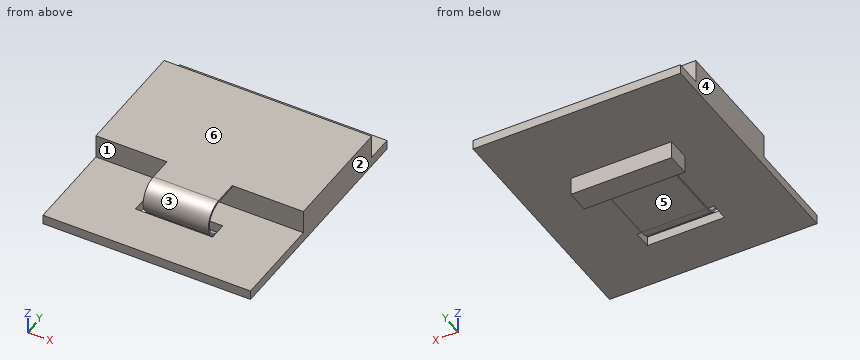
from build123d import *

# Parameters (mm, degrees)
F0_W     = 35
F0_H     = 40
F0_W_2   = 13
F0_H_2   = 3
F1_DEPTH = 1.6
F2_W     = 11
F2_H     = 1
F3_DEPTH = 4
F5_W     = 11
F5_H     = 0.3
F7_W     = 17
F7_H     = 3.9
F8_DEPTH = 3


with BuildPart() as f1:
    # F0 (on Top) → F1 (new body)
    with BuildSketch(Plane.XY):
        Rectangle(F0_W, F0_H)
        with Locations((0, -10.5)):
            Rectangle(F0_W_2, F0_H_2, mode=Mode.SUBTRACT)
    extrude(amount=F1_DEPTH)

    # F2 (on face) → F3 (join)
    with BuildSketch(Plane.XY.offset(1.6)):
        Polygon((17.5, 15.5), (-17.5, 15.5), (-17.5, -4.5), (-5.5, -4.5), (-5.5, -3.5), (5.5, -3.5), (5.5, -4.5), (17.5, -4.5), align=None)
        with Locations((0, -4)):
            Rectangle(F2_W, F2_H)
    extrude(amount=F3_DEPTH)

    # F6: sweep along a path in F4
    with BuildLine(Plane.YZ) as f6_path:
        Line((-4.5, 5.6), (-8.5, 5.6))
        ThreePointArc((-8.5, 5.6), (-11.5, 2.6), (-8.5, -0.4))
        Line((-8.5, -0.4), (6.975, -0.4))
    # F5 (on face) → F6 (sweep)
    with BuildSketch(Plane.XZ.offset(4.5)):
        with Locations((0, 5.45)):
            Rectangle(F5_W, F5_H)
    sweep(path=f6_path.line)

    # F7 (on face) → F8 (join)
    with BuildSketch(Plane(origin=(0, 0, 0), x_dir=(1, 0, 0), z_dir=(0, 0, -1))):
        with Locations((0, -5.025)):
            Rectangle(F7_W, F7_H)
    extrude(amount=F8_DEPTH)


solid = f1.part
Could you check a few things on this model? Use its own coordinates, in mm. Face numbers are marked on the shaded views. A direction names the side the tool comes from. Coordinates: 2 decimals unless noted, no trailing zeros. Order: outer loops, then holes, each group sorted by start corner. A loop starts at its lowest first (then second) coordinate and runs counter-clockwise, first axis right, second up. Notation, with made-up numbers: (23.25, 43) - (30.25, 43) arc R21 ccw to (30.25, 67) - close; hole circle Ø5 at (-13.5, 56). An arc over 180 degrees is marked (long way). Answer in a Markdown table with one row per item. Add a question column.
(1) If we section it at A-A, the plane z = 2.6: Please give me the cut outline in (x, y).
(2) If we section it at B-B, the plane x = -1: Please give me the cut outline in (y, z) (3 decimals).
(3) If we mould it in two halves opening along X, with no side actions, what happens to the marked faces 1, 2, 3 and 4? For each: released by +X, released by -X, zero draft, split by the parting line, or undercut.
(4) On a 3-axis mill with a long thin cutter (end or side, diameter ignored), from which of +Z, -Z, +X, -X, +Y, -Y can I reach the whole of each face in a straight line? I mean the marked faces 5 and 6. Say none if no direction works.
(5) Will these pins go through, and if not, where does the flat tip stop? pin 1 (3.5 mm diameter, centred on x = 2, z = -2, fed in from +Y) (3 decimals); pin 2 (0.9 mm diameter, centred on x = -1.5, z = -1.5, fed in from -Y) (3 decimals); pin 3 (2.5 mm diameter, centred on y = 5, z = -1.5, fed in from +X).
(6) I need wall thicknesses on L1, parallel to Y at x = 7, z = -0.5 (3 decimals); L2, parallel to Y at x = -4, z = 0.5; L3, parallel to Y at x = 12.5, z = 2. Which ranges of each line are inside material? Lowest first, please.
(7) If we section it at D-D, the plane x = 10: Please give me the cut outline in (y, z).
(8) If we section it at C-C, the plane z = 0.5: Please give me the cut outline in (x, y).
Results are:
| question | item | result |
|---|---|---|
| 1 | outline | (-17.5, -4.5) - (17.5, -4.5) - (17.5, 15.5) - (-17.5, 15.5) - close; (-5.5, -11.5) - (5.5, -11.5) - (5.5, -11.2) - (-5.5, -11.2) - close |
| 2 | outline | (-20, 0) - (-12, 0) - (-12, 1.6) - (-20, 1.6) - close; (-8.5, -0.4) - (3.075, -0.4) - (3.075, -3) - (6.975, -3) - (6.975, 0) - (20, 0) - (20, 1.6) - (15.5, 1.6) - (15.5, 5.6) - (-8.5, 5.6) arc R3 ccw to start; hole (-9, 0) - (-9, 1.6) - (-4.5, 1.6) - (-4.5, 5.3) - (-8.5, 5.3) arc R2.7 ccw to (-8.5, -0.1) - (3.075, -0.1) - (3.075, 0) - close |
| 3 | face 1 | zero draft |
| 3 | face 2 | released by +X |
| 3 | face 3 | undercut |
| 3 | face 4 | released by -X |
| 4 | face 5 | -Z, +X, -X, -Y |
| 4 | face 6 | +Z, +X, -X, +Y, -Y |
| 5 | pin 1 | stops at y = 6.975 |
| 5 | pin 2 | stops at y = 3.075 |
| 5 | pin 3 | stops at x = 8.5 |
| 6 | L1 | y = 3.075 to 6.975 |
| 6 | L2 | y = -20 to -12, -10.64 to -10.2, -9 to 20 |
| 6 | L3 | y = -4.5 to 15.5 |
| 7 | outline | (-20, 0) - (20, 0) - (20, 1.6) - (15.5, 1.6) - (15.5, 5.6) - (-4.5, 5.6) - (-4.5, 1.6) - (-20, 1.6) - close |
| 8 | outline | (-17.5, -20) - (17.5, -20) - (17.5, 20) - (-17.5, 20) - close; (-5.5, -10.64) - (5.5, -10.64) - (5.5, -10.2) - (-5.5, -10.2) - close; hole (-6.5, -12) - (6.5, -12) - (6.5, -9) - (-6.5, -9) - close |
